Geometry: see drawing. Coordinates: mm, zero at the bounding-box minimum. A direction names the side the tool comes from. Give positions to 0.01 mm unless a question says otherwise; leave off trailing zeros. Write each loop counter-clockwise with the first axis right and the second up, starting at its lowest first coordinate (ties: lowest second). Pieces come first, ordered by that corner, then holes. Notation, with made-up numbers: (-2, 34) - (6, 34) arc R27 ccw to (6, 59) - close; hole circle Ø11 at (69, -23). An arc over 180 degrees is marked (long way). Use a Markdown table: item, result. Add a question column.
1. Set-up query: the marked faces 1 and 2. Return all of +Z, -Z, +X, -X, +Y, -Y with unobstructed straight access to the full face (end or side cutting, diameter ignored); none if empty.
2. Section query A-A, the plane x = 1.5. Return loops of the section in (y, z).
3. Material intervals for probe 1 along X at (y, z) = (2, 3.75) (1 decimal); probe 2 along Y at (x, z) = (6.25, 5.75); probe 3 along X at (y, z) = (20, 3.5), sorted ascending.
4. Section query C-C, the plane y = 5.5. Return loops of the section in (x, z).
5. Section query D-D, the plane y = 23. Return loops of the section in (x, z), plus the area to 3 significant figures.
6. Pin query (flat end, axial travel): pin 1 (1 mm diameter, centred on x = 2.5, y = 4.5, fed in from +Z); pin 2 (2 mm diameter, centred on x = 3.5, y = 21.5, fed in from -Z); pin 3 (4 mm diameter, centred on y = 11, z = 6.5, fed in from +X). Return the tip coordinate at first contact, or that it passes through.
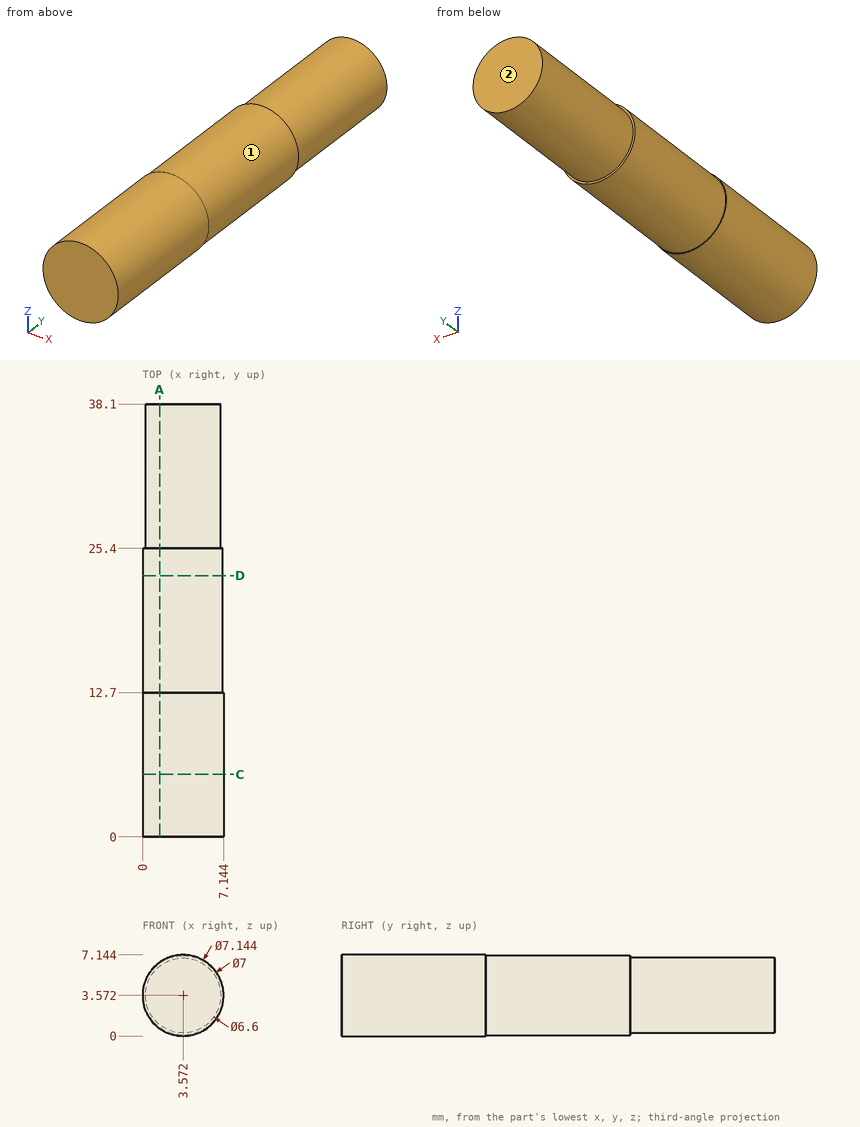
Result sheet:
| question | item | result |
|---|---|---|
| 1 | face 1 | +Y |
| 1 | face 2 | +Z, -Z, +X, -X, +Y |
| 2 | outline | (0, 0.66) - (12.7, 0.66) - (12.7, 0.75) - (25.4, 0.75) - (25.4, 1) - (38.1, 1) - (38.1, 6.14) - (25.4, 6.14) - (25.4, 6.39) - (12.7, 6.39) - (12.7, 6.48) - (0, 6.48) - close |
| 3 | probe 1 | x = 0 to 7.1 |
| 3 | probe 2 | y = 0 to 25.4 |
| 3 | probe 3 | x = 0.07 to 7.07 |
| 4 | outline | circle Ø7.14 at (3.57, 3.57) |
| 5 | outline | circle Ø7 at (3.57, 3.57) |
| 5 | area | 38.5 mm² |
| 6 | pin 1 | stops at z = 7.1 |
| 6 | pin 2 | stops at z = 0.07 |
| 6 | pin 3 | stops at x = 7.02 |
